Part print with two shaded views. Sizes in mm from the minimum x, y, z corner. A direction names the side the tool comes from. Round coordinates to 2 decimals unless told otherwise and drop trailing zeros. Write each loop counter-clockwise with the first axis right and the second up, starting at its lowest first coordinate (ties: lowest second). Pieces come first, ordered by that corner, then holes. Notation, with made-up numbers: (-33, 11) -> (-25, 11) arc R20 cw to (-25, 23) -> close; hole circle Ø5 at (26.5, 82.25). An arc over 180 degrees is marked (long way). Answer in a Markdown table with one row per item.
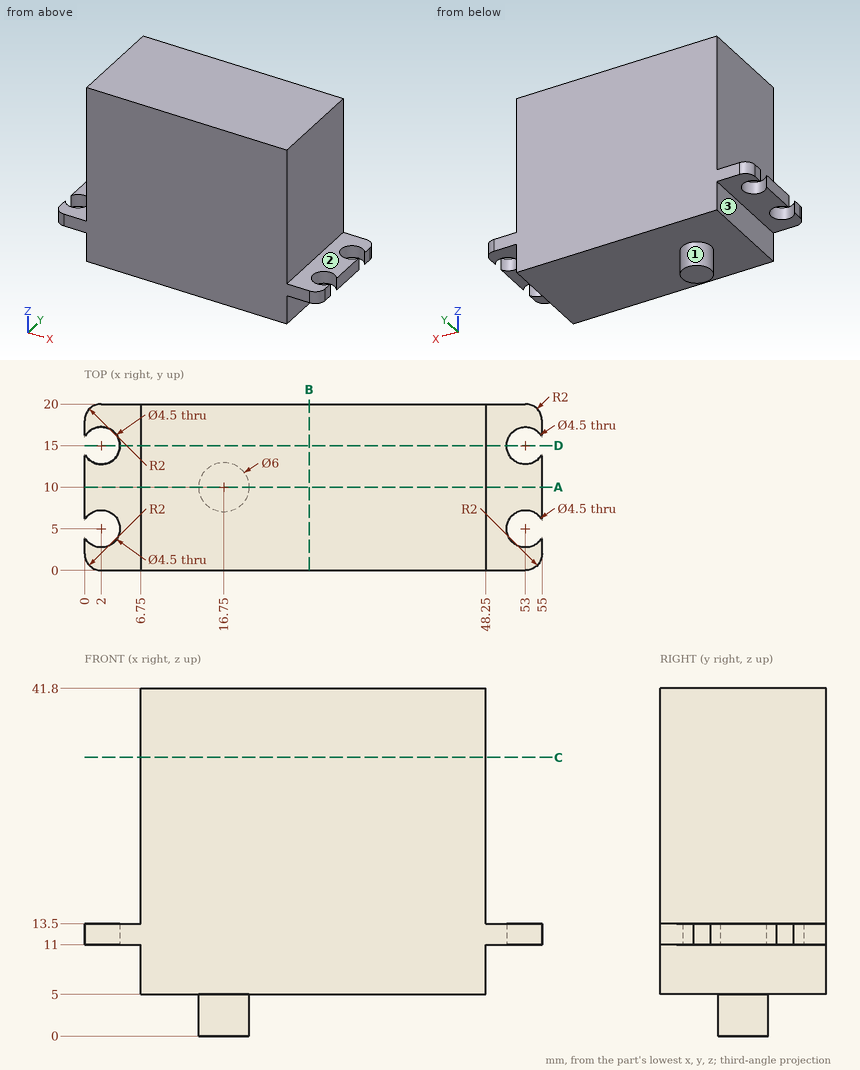
Q1. Wall check: line 1 (X direction, y = 16, z = 25); line 2 (Z direction, x = 37, y = 5); line 3 (Z direction, x = 49, y = 10). Give the ranges that are in metal, low to high. Write a range as [from, to].
A:
| item | result |
|---|---|
| line 1 | [6.75, 48.25] |
| line 2 | [5, 41.8] |
| line 3 | [11, 13.5] |
Q2. Saw through at D-D on y = 15. Write the cut outline in (x, z), plus the area to 3 significant figures.
A:
| item | result |
|---|---|
| outline | (4.25, 11) -> (6.75, 11) -> (6.75, 5) -> (48.25, 5) -> (48.25, 11) -> (50.75, 11) -> (50.75, 13.5) -> (48.25, 13.5) -> (48.25, 41.8) -> (6.75, 41.8) -> (6.75, 13.5) -> (4.25, 13.5) -> close |
| area | 1,540 mm² |
Q3. Which spindle directions (+Z, -Z, +X, -X, +Y, -Y) get a long thin tool onto all of the face, cutting with end or side? Do the marked faces 1, 2 and 3. Say none if no direction does.
A:
| item | result |
|---|---|
| face 1 | -Z |
| face 2 | +Z, +X, +Y, -Y |
| face 3 | -Z, -X, +Y, -Y |
Q4. Drop flat-ended pins along their axis: P1, Ø5, axis at y = 15, z = 20, coming from the +X side; P2, Ø6, axis at x = 2, y = 15, coming from the -Z side; P3, Ø4, axis at x = 53, y = 5, coming from the -Z side; P4, Ø2, axis at x = 2.5, y = 9.5, coming from the +Z side. Give the stop position or say it passes through.
A:
| item | result |
|---|---|
| P1 | x = 48.25 |
| P2 | z = 11 |
| P3 | through |
| P4 | z = 13.5 |
Q5. Saw through at A-A on y = 10. Write the cut outline in (x, z).
A:
| item | result |
|---|---|
| outline | (0, 11) -> (6.75, 11) -> (6.75, 5) -> (13.75, 5) -> (13.75, 0) -> (19.75, 0) -> (19.75, 5) -> (48.25, 5) -> (48.25, 11) -> (55, 11) -> (55, 13.5) -> (48.25, 13.5) -> (48.25, 41.8) -> (6.75, 41.8) -> (6.75, 13.5) -> (0, 13.5) -> close |
Q6. Saw through at B-B on x = 27. Write the cut outline in (y, z).
A:
| item | result |
|---|---|
| outline | (0, 5) -> (20, 5) -> (20, 41.8) -> (0, 41.8) -> close |
Q7. Saw through at C-C on z = 33.5. Write the cut outline in (x, y).
A:
| item | result |
|---|---|
| outline | (6.75, 0) -> (48.25, 0) -> (48.25, 20) -> (6.75, 20) -> close |
